Here's how the part is built. I have some questions about the finished solid (model axes, mm). Coordinates: 2 decimals unless noted, no trailing zeros. Write each loop counter-clockwise with the first axis right and the second up, starting at its lowest first coordinate (ties: lowest second). Pieces come first, ordered by that corner, then holes. Notation, with made-up numbers: (35.25, 53.5) -> (39.25, 53.5) arc R28 ccw to (39.25, 80.5) -> close; hole circle Ø9 at (17.5, -30.5). An arc over 180 degrees is marked (long way). Put each result on its own line as item: value.
```python
from build123d import *

# Parameters (mm, degrees)
SKETCH1_R           = 1.75
BOSS_EXTRUDE1_DEPTH = 4


with BuildPart() as part:
    # Sketch1 → Boss-Extrude1 (new body)
    with BuildSketch(Plane.XY):
        with BuildLine():
            Line((163.58008547, 21.295659048), (163.58008547, 47.795659048))
            ThreePointArc((163.58008547, 47.795659048), (164.165871907, 49.209872611), (165.58008547, 49.795659048))
            Line((165.58008547, 49.795659048), (178.58008547, 49.795659048))
            ThreePointArc((178.58008547, 49.795659048), (179.287192251, 50.088552267), (179.58008547, 50.795659048))
            Line((179.58008547, 50.795659048), (179.58008547, 52.795659048))
            ThreePointArc((179.58008547, 52.795659048), (179.287192251, 53.502765829), (178.58008547, 53.795659048))
            Line((178.58008547, 53.795659048), (64.58008547, 53.795659048))
            ThreePointArc((64.58008547, 53.795659048), (63.872978688, 53.502765829), (63.58008547, 52.795659048))
            Line((63.58008547, 52.795659048), (63.58008547, 50.795659048))
            ThreePointArc((63.58008547, 50.795659048), (63.872978688, 50.088552267), (64.58008547, 49.795659048))
            Line((64.58008547, 49.795659048), (77.58008547, 49.795659048))
            ThreePointArc((77.58008547, 49.795659048), (78.994299032, 49.209872611), (79.58008547, 47.795659048))
            Line((79.58008547, 47.795659048), (79.58008547, 21.295659048))
            ThreePointArc((79.58008547, 21.295659048), (84.41282358, 9.628397159), (96.08008547, 4.795659048))
            Line((96.08008547, 4.795659048), (147.08008547, 4.795659048))
            ThreePointArc((147.08008547, 4.795659048), (158.747347359, 9.628397159), (163.58008547, 21.295659048))
        make_face()
        with Locations((89.03008547, 40.987963894)):
            Circle(SKETCH1_R, mode=Mode.SUBTRACT)
        with Locations((86.946454525, 12.162028103)):
            Circle(SKETCH1_R, mode=Mode.SUBTRACT)
        with Locations((154.12258547, 40.987963894)):
            Circle(SKETCH1_R, mode=Mode.SUBTRACT)
        with Locations((156.213716414, 12.162028103)):
            Circle(SKETCH1_R, mode=Mode.SUBTRACT)
    extrude(amount=BOSS_EXTRUDE1_DEPTH)


solid = part.part
```
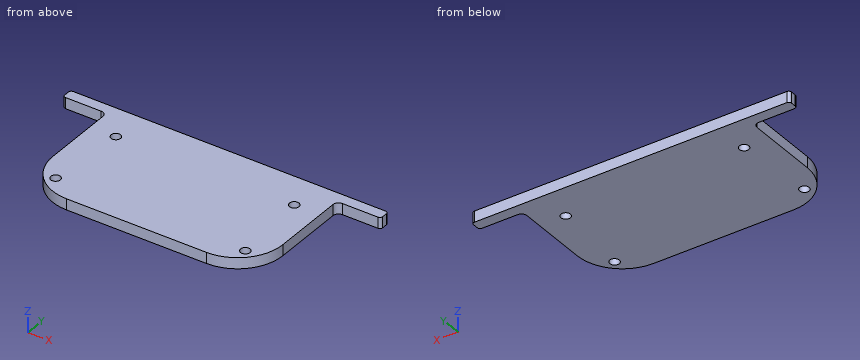
Item 1: Imagine slicing it at A-A on z = 0.7. Write out the boundary of the cut face in (x, y), then the cut area to 3 significant figures.
Output:
outline: (63.58, 50.8) arc R1 ccw to (64.58, 49.8) -> (77.58, 49.8) arc R2 cw to (79.58, 47.8) -> (79.58, 21.3) arc R16.5 ccw to (96.08, 4.8) -> (147.08, 4.8) arc R16.5 ccw to (163.58, 21.3) -> (163.58, 47.8) arc R2 cw to (165.58, 49.8) -> (178.58, 49.8) arc R1 ccw to (179.58, 50.8) -> (179.58, 52.8) arc R1 ccw to (178.58, 53.8) -> (64.58, 53.8) arc R1 ccw to (63.58, 52.8) -> close; hole circle Ø3.5 at (86.95, 12.16); hole circle Ø3.5 at (89.03, 40.99); hole circle Ø3.5 at (154.12, 40.99); hole circle Ø3.5 at (156.21, 12.16)
area: 4,090 mm²
Item 2: Imagine slicing it at B-B on y = 26.5. Write out the boundary of the cut face in (x, z).
Output:
outline: (79.58, 0) -> (163.58, 0) -> (163.58, 4) -> (79.58, 4) -> close
Item 3: For P1, Ø1.2, axis at x = 174.5, z = 1.5, coming from the -Y side; P2, Ø1.2, axis at y = 29.5, z = 3, coming from the +X side, each with a flat end and sliding along its axis, tell me the tip position at first contact or that it passes through.
Output:
P1: stops at y = 49.8
P2: stops at x = 163.58
Item 4: Please list where these lines run through material, in increasing order: line 1 along X through (y, z) = (44.5, 3.3); line 2 along X through (y, z) = (13.5, 2.6); line 3 along Y through (x, z) = (169.5, 1.7). Write a range as from..to.
Output:
line 1: x = 79.58..163.58
line 2: x = 81.54..85.82, 88.07..155.09, 157.34..161.62
line 3: y = 49.8..53.8
